Autodesk Inventor part; units mm, degrees
ref_plane "YZ Plane" through (0, 0, 0) normal (1, 0, 0) x (0, 1, 0)
ref_plane "XZ Plane" through (0, 0, 0) normal (0, 1, 0) x (-1, 0, 0)
ref_plane "XY Plane" through (0, 0, 0) normal (0, 0, 1) x (1, 0, 0)
sketch "Sketch13" plane through (0, 0, 0) normal (0, 0, 1) x (1, 0, 0)
  line L0 (-25, 12.5) -> (25, 12.5)
  line L1 (25, 12.5) -> (25, -12.5)
  line L2 (25, -12.5) -> (-25, -12.5)
  line L3 (-25, -12.5) -> (-25, 12.5)
  line L4 (-25, 12.5) -> (25, -12.5) construction
  line L5 (25, 12.5) -> (-25, -12.5) construction
  point P0 (0, 0)
  dimension "d26" = 50
  dimension "d27" = 25
extrude "Extrusion14" add sketch "Sketch13" along normal blind 5
sketch "Sketch14" plane through (0, 0, 0) normal (0, 0, -1) x (-1, 0, 0)
  line L0 (25, -12.5) -> (-25, -12.5)
  line L1 (25, 12.5) -> (25, -12.5)
  line L2 (-25, 12.5) -> (25, 12.5)
  line L3 (-25, -12.5) -> (-25, 12.5)
  line L4 (-25, -12.5) -> (-25, 12.5)
  line L5 (-25, 2.5) -> (25, 2.5)
  line L6 (25, 12.5) -> (25, -12.5)
  point P0 (0, 0)
  point P1 (25, 2.5)
  dimension "d30" = 10
extrude "Extrusion15" cut sketch "Sketch14" against normal blind 3 contours L5 L3 L2 L1
sketch "Sketch16" plane through (0, 0, 3) normal (0, 0, -1) x (-1, 0, 0)
  line L0 (-25, 2.5) -> (-25, 12.5)
  line L1 (25, 2.5) -> (-25, 2.5)
  line L2 (25, 12.5) -> (25, 2.5)
  line L3 (-25, 12.5) -> (25, 12.5)
  point P0 (0, 0)
  point P1 (-15, 7.5)
  point P2 (15, 7.5)
  point P3 (-25, 7.5)
  point P4 (25, 7.5)
  dimension "d33" = 10
  dimension "d34" = 10
hole "Hole1" at (15, 7.5, 3) at (-15, 7.5, 3) direction (0, 0, 1) diameter 2.9 end through all
sketch "Sketch17" plane through (0, 0, 5) normal (0, 0, 1) x (1, 0, 0)
  line L0 (-25, 12.5) -> (-25, -12.5)
  line L1 (25, -12.5) -> (25, 12.5)
  point P0 (0, 0)
  point P1 (-15, -5)
  point P2 (15, -5)
  dimension "d42" = 7.5
  dimension "d43" = 10
  dimension "d44" = 10
hole "Hole2" at (-15, -5, 5) at (15, -5, 5) direction (0, 0, -1) diameter 3.2 end through all
properties part number "Beam Cover Bracket" material "ABS Plastic"
Geometry: final body of the model. Coordinates: model frame, mm. A direction names the side the tool comes from. Round coordinates to 2 decimals unless told otherwise and drop trailing zeros. Order: outer loops, then holes, each group sorted by start corner. A loop starts at its lowest first (then second) coordinate and runs counter-clockwise, first axis right, second up. Notation, with made-up numbers: (-0.5, 52) -> (38.5, 52) arc R11 ccw to (38.5, 70) -> close; hole circle Ø7 at (23.25, 81.5). An arc over 180 degrees is marked (long way). Write each question's results on one line, items separated by ' | '.
Q1. Pin query (flat end, axial travel): pin 1 Ø0.9 at (x, z) = (-9.5, 1) entering from +Y. Return the tip coordinate at first contact, or that it passes through.
Response values:
pin 1: y = 2.5
Q2. Section query C-C (z = 2.4). Output: boundary loops of the cut face in (x, y), and give its area (3 significant figures).
Response values:
outline: (-25, -12.5) -> (25, -12.5) -> (25, 2.5) -> (-25, 2.5) -> close; hole circle Ø3.2 at (-15, -5); hole circle Ø3.2 at (15, -5) | area: 734 mm²
Q3. Section query D-D (y = -5). Output: boundary loops of the cut face in (x, z), and give its area (3 significant figures).
Response values:
outline: (-25, 0) -> (-16.6, 0) -> (-16.6, 5) -> (-25, 5) -> close; (-13.4, 0) -> (13.4, 0) -> (13.4, 5) -> (-13.4, 5) -> close; (16.6, 0) -> (25, 0) -> (25, 5) -> (16.6, 5) -> close | area: 218 mm²
Q4. Pull-direction query (Y, two-part tool) for faces 1 (the face through (0, 12.5, 4)), 2 (the face through (14.94, 6.05, 4.01)), 3 (the face through (0, 8, 3)), 4 (the face through (0, -12.5, 2)); classes: released by +Y, released by -Y, zero draft, split by the parting line, or undercut.
Response values:
face 1: released by +Y | face 2: undercut | face 3: zero draft | face 4: released by -Y
Q5. Access query for faces 5 (the face through (0, 0, 5)), 6 (the face through (0, 2.5, 1)). Directions: +Z, -Z, +X, -X, +Y, -Y. A direction counts if a zero-diameter tool reaches every point of the face in a straight line with its end or side. Return the directions, or none.
Response values:
face 5: +Z, +X, -X, +Y, -Y | face 6: -Z, +X, -X, +Y
Q6. Ray query, line 1 along X through (y, z) = (-5, 2.45); line 2 along X through (y, z) = (7.5, 3.75); line 3 along Y through (x, z) = (-15, 3.1). Return the intervals inside material, ascending.
Response values:
line 1: -25 to -16.6, -13.4 to 13.4, 16.6 to 25 | line 2: -25 to -16.45, -13.55 to 13.55, 16.45 to 25 | line 3: -12.5 to -6.6, -3.4 to 6.05, 8.95 to 12.5
Q7. Section query B-B (y = 7.5). Output: boundary loops of the cut face in (x, z), and give its area (3 significant figures).
Response values:
outline: (-25, 3) -> (-16.45, 3) -> (-16.45, 5) -> (-25, 5) -> close; (-13.55, 3) -> (13.55, 3) -> (13.55, 5) -> (-13.55, 5) -> close; (16.45, 3) -> (25, 3) -> (25, 5) -> (16.45, 5) -> close | area: 88.4 mm²
Q8. Section query A-A (x = 15). Output: boundary loops of the cut face in (y, z).
Response values:
outline: (-12.5, 0) -> (-6.6, 0) -> (-6.6, 5) -> (-12.5, 5) -> close; (-3.4, 0) -> (2.5, 0) -> (2.5, 3) -> (6.05, 3) -> (6.05, 5) -> (-3.4, 5) -> close; (8.95, 3) -> (12.5, 3) -> (12.5, 5) -> (8.95, 5) -> close
